```python
from build123d import *

# Parameters (mm, degrees)
SKETCH1_R           = 1.5
BOSS_EXTRUDE1_DEPTH = 4.3
SKETCH2_W           = 89
SKETCH2_H           = 54
BOSS_EXTRUDE2_DEPTH = 80


with BuildPart() as part:
    # Sketch1 → Boss-Extrude1 (new body)
    with BuildSketch(Plane(origin=(0, 0, 0), x_dir=(1, 0, 0), z_dir=(0, 1, 0))):
        Polygon((-35.5, 27), (-35.5, 33), (-55, 33), (-55, -33), (55, -33), (55, 33), (35.5, 33), (35.5, 27), (15.5, 27), (15.5, 33), (-15.5, 33), (-15.5, 27), align=None)
        with Locations(Location((-42.2, -30.2, 0), (0, 0, 90))):
            Circle(SKETCH1_R, mode=Mode.SUBTRACT)
        with Locations(Location((-50.2, -23.1, 0), (0, 0, 90))):
            Circle(SKETCH1_R, mode=Mode.SUBTRACT)
        with Locations(Location((-42.2, -24.2, 0), (0, 0, 90))):
            Circle(SKETCH1_R, mode=Mode.SUBTRACT)
        with Locations(Location((42.2, -30.2, 0), (0, 0, 90))):
            Circle(SKETCH1_R, mode=Mode.SUBTRACT)
        with Locations(Location((42.2, -24.2, 0), (0, 0, 90))):
            Circle(SKETCH1_R, mode=Mode.SUBTRACT)
        with Locations(Location((50.2, -23.1, 0), (0, 0, 90))):
            Circle(SKETCH1_R, mode=Mode.SUBTRACT)
        with Locations(Location((-50.2, 17.5, 0), (0, 0, 90))):
            Circle(SKETCH1_R, mode=Mode.SUBTRACT)
        with Locations(Location((-42.2, 18.5, 0), (0, 0, 90))):
            Circle(SKETCH1_R, mode=Mode.SUBTRACT)
        with Locations(Location((-42.2, 24.5, 0), (0, 0, 90))):
            Circle(SKETCH1_R, mode=Mode.SUBTRACT)
        with Locations(Location((42.2, 18.5, 0), (0, 0, 90))):
            Circle(SKETCH1_R, mode=Mode.SUBTRACT)
        with Locations(Location((50.2, 17.5, 0), (0, 0, 90))):
            Circle(SKETCH1_R, mode=Mode.SUBTRACT)
        with Locations(Location((42.2, 24.5, 0), (0, 0, 90))):
            Circle(SKETCH1_R, mode=Mode.SUBTRACT)
    extrude(amount=BOSS_EXTRUDE1_DEPTH)

    # Sketch2 → Boss-Extrude2 (add)
    with BuildSketch(Plane(origin=(0, 4.3, 0), x_dir=(1, 0, 0), z_dir=(0, 1, 0))):
        Rectangle(SKETCH2_W, SKETCH2_H)
    extrude(amount=BOSS_EXTRUDE2_DEPTH)


solid = part.part
```
CAD build for the part. Positions are in the model's coordinates, mm. A direction names the side the tool comes from. Round coordinates to 2 decimals unless told otherwise and drop trailing zeros. Loops run counter-clockwise (first coordinate to the right, second up) from the corner with the lowest first, then second, coordinate; pieces in that order, holes last. Notation, with made-up numbers: (-13, 31) - (31, 31) arc R24 ccw to (31, 61) - close; hole circle Ø10 at (5, 70.25). An arc over 180 degrees is marked (long way). Return JSON: item names as keys, results as strings. Group by question number.
Q1. Band-saw the part on C-C on z = 13. Give the cut face in (x, y).
Q2. Band-saw the part on A-A on z = 30.2. Give the cut face in (x, y).
Q3. Tool access for faces 4 (the face through (-55, 2, 0)), 5 (the face through (0, 4.3, -30)), 6 (the face through (35.5, 2, -30)), 7 (the face through (42, 4.3, -25)): list every direction of +Z, -Z, +X, -X, +Y, -Y with a clear straight run to the whole face (end or side of a thin tool).
Q4. Two-plate mould, pull along Z, no slides. Class faces 1 (the face through (-45, 2, -33)), 2 (the face through (-42, 4.3, 24)), 3 (the face through (15.5, 2, -30)): +Z half, -Z half, draft (parallel to the pull), parting line (faces both ways), or undercut.
Q5. Drill centre lines: line 1 along Z through (x, y) = (-42.2, 3.35); line 2 along Z through (x, y) = (50, 3); line 3 along X through (y, z) = (1.45, -17.5). Where is each one in solid material? Low to high. Write a range as [from, to].
Q6. Flat gauge pins, fed straight in: pin 1 Ø24 at (x, y) = (15, 60.5) entering from +Z; pin 2 Ø2.5 at (x, z) = (42.2, -18.5) entering from -Y; pin 3 Ø3.5 at (x, z) = (-50.2, 23.1) entering from +Y; pin 4 Ø2.5 at (x, z) = (-41.5, -24.5) entering from -Y. Where does each tip first touch, or does it go through?
Q7. Band-saw the part on D-D on y = 46. Give the cut face in (x, z), plus the area to 3 significant figures.
Q8. Band-saw the part on B-B on x = 12. Give the cut face in (y, z), plus the area to 3 significant figures.
Solutions:
{
 "1": {"outline": "(-55, 0) - (55, 0) - (55, 4.3) - (44.5, 4.3) - (44.5, 84.3) - (-44.5, 84.3) - (-44.5, 4.3) - (-55, 4.3) - close"},
 "2": {"outline": "(-55, 0) - (-43.7, 0) - (-43.7, 4.3) - (-55, 4.3) - close; (-40.7, 0) - (40.7, 0) - (40.7, 4.3) - (-40.7, 4.3) - close; (43.7, 0) - (55, 0) - (55, 4.3) - (43.7, 4.3) - close"},
 "3": {"face 4": "+Z, -Z, -X, +Y, -Y", "face 5": "-Z, +X, -X, +Y", "face 6": "-Z, +Y, -Y", "face 7": "-Y"},
 "4": {"face 1": "-Z half", "face 2": "undercut", "face 3": "draft"},
 "5": {"line 1": "z = [-33, -26], [-23, -20], [-17, 22.7], [25.7, 28.7], [31.7, 33]", "line 2": "z = [-33, -18.99], [-16.01, 21.61], [24.59, 33]", "line 3": "x = [-55, -51.7], [-48.7, -43.32], [-41.08, 41.08], [43.32, 48.7], [51.7, 55]"},
 "6": {"pin 1": "stops at z = 27", "pin 2": "stops at y = 4.3", "pin 3": "stops at y = 4.3", "pin 4": "stops at y = 0"},
 "7": {"outline": "(-44.5, -27) - (44.5, -27) - (44.5, 27) - (-44.5, 27) - close", "area": "4,810 mm^2"},
 "8": {"outline": "(0, -33) - (4.3, -33) - (4.3, -27) - (84.3, -27) - (84.3, 27) - (4.3, 27) - (4.3, 33) - (0, 33) - close", "area": "4,600 mm^2"}
}
